from build123d import *

# Parameters (mm, degrees)
F1_DEPTH = 70
F2_R     = 4
F3_DEPTH = 50


with BuildPart() as f1:
    # F0 (on Top) → F1 (new body)
    with BuildSketch(Plane.XY):
        with BuildLine():
            Line((53.26148, 34.026845), (-61.73852, 34.026845))
            Line((-61.73852, 34.026845), (-61.73852, 24.026845))
            Line((-61.73852, 24.026845), (43.26148, 24.026845))
            ThreePointArc((43.26148, 24.026845), (46.797014, 22.562379), (48.26148, 19.026845))
            Line((48.26148, 19.026845), (48.26148, -10.973155))
            ThreePointArc((48.26148, -10.973155), (46.797014, -14.508688), (43.26148, -15.973155))
            Line((43.26148, -15.973155), (-61.73852, -15.973155))
            Line((-61.73852, -15.973155), (-61.73852, -25.973155))
            Line((-61.73852, -25.973155), (53.26148, -25.973155))
            ThreePointArc((53.26148, -25.973155), (56.797014, -24.508688), (58.26148, -20.973155))
            Line((58.26148, -20.973155), (58.26148, 29.026845))
            ThreePointArc((58.26148, 29.026845), (56.797014, 32.562379), (53.26148, 34.026845))
        make_face()
    extrude(amount=F1_DEPTH)

    # F2 (on face) → F3 (join, through all)
    with BuildSketch(Plane.XZ.offset(25.973155)):
        with Locations((-4.23852, 35)):
            Circle(F2_R)
    extrude(amount=-F3_DEPTH)


solid = f1.part
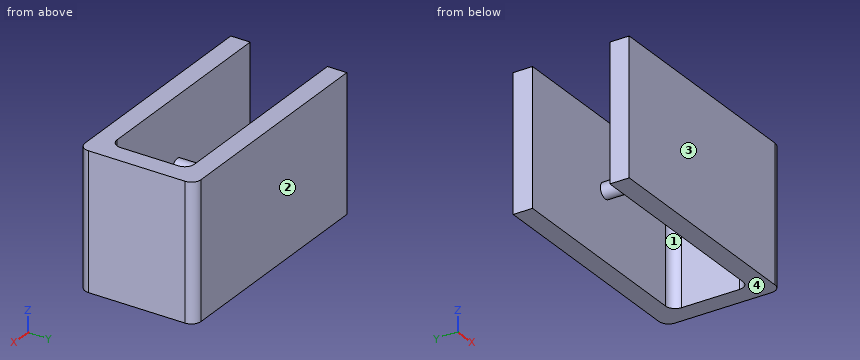
Could you check a few things on this model? Use its own coordinates, in mm. Face numbers are marked on the shaded views. Give positions to 0.01 mm unless a question says otherwise; leave off trailing zeros. Order: outer loops, then holes, each group sorted by start corner. A loop starts at its lowest first (then second) coordinate and runs counter-clockwise, first axis right, second up.
1. Thinking about a two-plate mould opening in Y: for the marked faces 1, 2, 3 and 4, which applies, +Y half, -Y half, draft (parallel to the pull), parting line (faces both ways), or undercut?
Answers below:
face 1: undercut
face 2: +Y half
face 3: -Y half
face 4: draft
2. Suppose I cut it at A-A (y = -8). Write out the boundary of the cut face in (x, z), plus the area to 3 significant figures.
Answers below:
outline: circle Ø8 at (-4.24, 35); (48.26, 0) - (58.26, 0) - (58.26, 70) - (48.26, 70) - close
area: 750 mm2
3. Suppose I cut it at D-D (z = 43). Write out the boundary of the cut face in (x, y).
Answers below:
outline: (-61.74, -25.97) - (53.26, -25.97) arc R5 ccw to (58.26, -20.97) - (58.26, 29.03) arc R5 ccw to (53.26, 34.03) - (-61.74, 34.03) - (-61.74, 24.03) - (43.26, 24.03) arc R5 cw to (48.26, 19.03) - (48.26, -10.97) arc R5 cw to (43.26, -15.97) - (-61.74, -15.97) - close
4. I need wall thicknesses on L1, parallel to Y at x = 34, z = 26; L2, parallel to X at y = 19, z = 39.5; L3, parallel to X at y = 7.5, z = 38. Which ranges of each line are inside material? Lowest first, please.
Answers below:
L1: y = -25.97 to -15.97, 24.03 to 34.03
L2: x = 48.26 to 58.26
L3: x = -6.88 to -1.59, 48.26 to 58.26
5. Suppose I cut it at B-B (x = -45). Write out the boundary of the cut face in (y, z), plus the area to 3 significant figures.
Answers below:
outline: (-25.97, 0) - (-15.97, 0) - (-15.97, 70) - (-25.97, 70) - close; (24.03, 0) - (34.03, 0) - (34.03, 70) - (24.03, 70) - close
area: 1,400 mm2
6. For pin 1 (3 mm diameter, centred on y = 7, z = 46, fed in from -X); pin 2 (6 mm diameter, centred on x = -30.5, y = 19.5, fed in from +Z); pin 3 (1.5 mm diameter, centred on x = -4, y = 19, fed in from +Z), each with a flat end and sliding along its axis, tell me the tip position at first contact or that it passes through.
Answers below:
pin 1: stops at x = 48.26
pin 2: passes through
pin 3: stops at z = 39
7. Suppose I cut it at C-C (z = 35). Write out the boundary of the cut face in (x, y), plus the area to 3 significant figures.
Answers below:
outline: (-61.74, -25.97) - (53.26, -25.97) arc R5 ccw to (58.26, -20.97) - (58.26, 29.03) arc R5 ccw to (53.26, 34.03) - (-61.74, 34.03) - (-61.74, 24.03) - (-8.24, 24.03) - (-8.24, -15.97) - (-61.74, -15.97) - close; hole (-0.24, -15.97) - (43.26, -15.97) arc R5 ccw to (48.26, -10.97) - (48.26, 19.03) arc R5 ccw to (43.26, 24.03) - (-0.24, 24.03) - close
area: 3,120 mm2
